Autodesk Inventor part; units mm, degrees
ref_plane "Work Plane1" through (-17.387, -14.1299, -4.1299) normal (1, 0, 0) x (0, 1, 0)
ref_plane "YZ Plane" through (0, 0, 0) normal (1, 0, 0) x (0, 1, 0)
ref_plane "XZ Plane" through (0, 0, 0) normal (0, 1, 0) x (-1, 0, 0)
sketch "Sketch1" plane through (0, 0, 0) normal (1, 0, 0) x (0, 1, 0)
  line L0 (9.9, 0) -> (6.6104, -37.6)
  line L1 (11, 0) -> (11, -20)
  line L2 (-11, 0) -> (11, 0)
  line L3 (8.722, -6.7025) -> (0, -6.7025)
  line L4 (0, -6.7025) -> (0, 40.232)
  line L5 (0, 40.232) -> (3.984, 40.232)
  line L6 (3.984, 40.232) -> (11, 0) construction
  arc A0 (6.0149, 28.5859) -> (5.3277, 32.5264) centre (2.2587, 29.961) ccw construction
  line L7 (3.984, 40.232) -> (11.8979, 22.8363)
  line L8 (11.8979, 22.8363) -> (11.8979, 2.3768)
  line L9 (11.8979, 2.3768) -> (9.3084, 0)
  line L10 (9.3084, 0) -> (8.722, -6.7025)
  point P0 (0, 0)
  dimension "d4" = 4
  dimension "d5" = 4
revolve "Revolution1" add sketch "Sketch1" angle 360 about axis through (0, 0, -6.7025) along (0, 0, 1)
sketch "Sketch2" plane through (0, 0, 0) normal (1, 0, 0) x (0, 1, 0)
  line L0 (-3.984, 40.232) -> (-11.8979, 22.8363)
  line L1 (0, 39.9349) -> (0, 14.7253)
  arc A0 (-3.984, 40.232) -> (-3.4864, 41.3256) centre (-5.4716, 41.5688) ccw
  point P0 (0, 0)
  dimension "d7" = 2
sketch "Sketch3" plane through (0, 0, 0) normal (1, 0, 0) x (0, 1, 0)
  circle A0 centre (0, 10) radius 7.21
  circle A1 centre (0, 13.2675) radius 9.5
  point P0 (0, 0)
  dimension "d8" = 19
ref_plane "Work Plane1" through (-17.387, -14.1299, -4.1299) normal (1, 0, 0) x (0, 1, 0)
extrude "Extrusion1" add sketch "Sketch3" against normal up to surface (17.387 mm away) contours A0 A1 | A0 A1 picked at (-1.9464, 7.9731) picked at (-0.0449, 20.8614)
sketch "Sketch4" plane through (-17.387, 0, 13.2675) normal (-1, 0, 0) x (0, 0, 1)
  circle A0 centre (0, 0) radius 9.5
  circle A1 centre (0, 0) radius 7.75
  point P0 (-13.2675, 0)
  dimension "d11" = 15.5
extrude "Extrusion2" cut sketch "Sketch4" against normal blind 15 contours A1
sketch "Sketch5" plane through (0, 0, -6.7025) normal (0, 0, -1) x (-1, 0, 0)
  circle A0 centre (0, 0) radius 9.3084
  circle A1 centre (0, 0) radius 7.2846
  point P0 (0, 0)
extrude "Extrusion3" cut sketch "Sketch5" against normal through all draft -5 contours A1
properties part number "01_Connector_T"
Verification items for the finished model (mm, model axes). A direction names the side the tool comes from. Coordinates: 2 decimals unless noted, no trailing zeros. Write each loop counter-clockwise with the first axis right and the second up, starting at its lowest first coordinate (ties: lowest second). Pieces come first, ordered by that corner, then holes. Notation, with made-up numbers: M 12.5,51 L 27.5,51 A12 cw 27.5,72 Z; hole C 32,1 d9. An arc over 180 degrees is marked long. Use a Markdown table: item, result.
Q1. Set-up check for faces 1 (the face through (8.74, -1.94, -4.05)), 2 (the face through (-2.387, 6, 14)): record each of +Z, -Z, +X, -X, +Y, -Y from which the full face is reachable in a straight line by a thin tool's end or side.
Reply:
| item | result |
|---|---|
| face 1 | -Z |
| face 2 | -X |
Q2. Sectioned sample at A-A, the plane y = 0. Record the boundary of the cut face in (x, z).
Reply:
| item | result |
|---|---|
| outline | M -17.39,3.77 L -11.9,3.77 L -11.9,2.38 L -9.31,0 L -8.72,-6.7 L -7.28,-6.7 L -6.22,5.52 L -17.39,5.52 Z; M -17.39,21.02 L -4.86,21.02 L -3.18,40.23 L -3.98,40.23 L -11.9,22.84 L -11.9,22.77 L -17.39,22.77 Z; M 3.18,40.23 L 7.28,-6.7 L 8.72,-6.7 L 9.31,0 L 11.9,2.38 L 11.9,22.84 L 3.98,40.23 Z |
Q3. Thickness scan on line 1 (Z direction, x = -14, y = 0); line 2 (Z direction, x = -10.5, y = 0); line 3 (Y direction, x = -8, z = 13). Record the ranges inside material, lowest first.
Reply:
| item | result |
|---|---|
| line 1 | z = 3.77 to 5.52, 21.02 to 22.77 |
| line 2 | z = 1.09 to 5.52, 21.02 to 25.91 |
| line 3 | y = -9.5 to -7.75, 7.75 to 9.5 |
Q4. Go/stop test with flat-tipped pins: P1, Ø1, axis at y = 6, z = 15, coming from the -X side; P2, Ø10, axis at y = 9, z = 1, coming from the -X side; P3, Ø3, axis at x = 0, z = 30.5, coming from the -Y side. Record where each tip stops, or that it passes through.
Reply:
| item | result |
|---|---|
| P1 | stops at x = -2.39 |
| P2 | stops at x = -11.13 |
| P3 | stops at y = -9.09 |
Q5. Sectioned sample at C-C, the plane z = 8.5. Record the boundary of the cut face in (x, y).
Reply:
| item | result |
|---|---|
| outline | M -17.39,-8.22 L -8.6,-8.22 A11.9 ccw long -8.6,8.22 L -17.39,8.22 L -17.39,6.11 L -2.39,6.11 L -2.39,5.46 A5.95 cw long -2.39,-5.46 L -2.39,-6.11 L -17.39,-6.11 Z |
Q6. Draft check along Y on faces 3 (the face through (-2.387, -6, 14)), 4 (the face through (9.25, -2.05, 0.15)), 5 (the face through (-17.387, -8, 13)). Enter one of: +Y half, -Y half, draft (parallel to the pull), parting line (faces both ways), or undercut.
Reply:
| item | result |
|---|---|
| face 3 | undercut |
| face 4 | parting line |
| face 5 | draft |
Q7. Sectioned sample at D-D, the plane z = 31.5. Record the boundary of the cut face in (x, y), plus the area to 3 significant figures.
Reply:
| item | result |
|---|---|
| outline | C 0,0 d15.91; hole C 0,0 d7.88 |
| area | 150 mm² |
Q8. Sectioned sample at B-B, the plane x = 0. Record the boundary of the cut face in (y, z), plus the area to 3 significant figures.
Reply:
| item | result |
|---|---|
| outline | M -11.9,2.38 L -9.31,0 L -8.72,-6.7 L -7.28,-6.7 L -3.18,40.23 L -3.98,40.23 L -11.9,22.84 Z; M 3.18,40.23 L 7.28,-6.7 L 8.72,-6.7 L 9.31,0 L 11.9,2.38 L 11.9,22.84 L 3.98,40.23 Z |
| area | 443 mm² |
